Source: three-view drawing plus pictorial views. Frame: mm from the lowest corner of the part. A direction names the side the tool comes from. Round coordinates to 2 decimals unless told otherwise and drop trailing zeros. Write each loop counter-clockwise with the first axis right and the second up, starting at its lowest first coordinate (ties: lowest second). Pieces come first, ordered by that corner, then holes. Notation, with made-up numbers: M -2,-5.5 L 49,-5.5 A24 cw 49,4.5 Z; hole C 51.5,-26 d5. An arc over 180 degrees is marked long. Put each result on its own line as item: value. Start each with the question number.
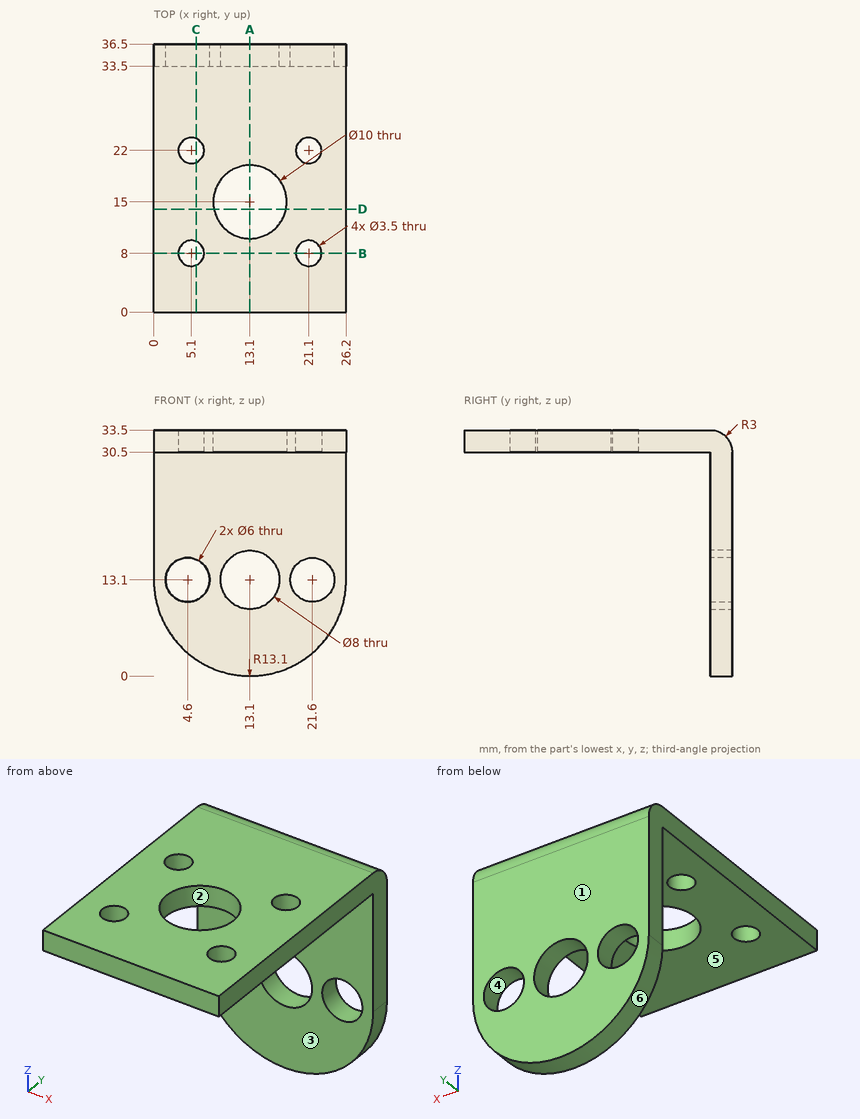
(1) Ray query, line 1 along Y through (x, z) = (18.25, 5.5); line 2 along Y through (x, z) = (5.1, 32.85); line 3 along Y through (x, z) = (5.1, 32.1). Return the intervals inside material, ascending.
(2) Access query for the marked faces 5 and 6. Directions: +Z, -Z, +X, -X, +Y, -Y. A direction counts if a zero-diameter tool reaches every point of the face in a straight line with its end or side. Return the directions, or none.
(3) Section query C-C (x = 5.75). Return loops of the section in (y, z).
(4) Pull-direction query (Y, two-part tool) for the marked faces 1, 2, 3 and 4; classes: +Y half, -Y half, draft (parallel to the pull), parting line (faces both ways), or undercut.
(5) Section query A-A (x = 13.1). Return loops of the section in (y, z).
(6) Contact query for flat-ended pins moving along their axis: P1, Ø5, axis at x = 8.5, z = 23, coming from the -Y side; P2, Ø2, axis at x = 22, z = 11.5, coming from the +Y side; P3, Ø4.5, axis at x = 21.1, y = 22, coming from the -Z side. Output: stop coordinate, or through.
(7) Section query B-B (y = 8). Return loops of the section in (x, z).
(8) Section query D-D (y = 14). Return loops of the section in (x, z), and give its area (3 significant figures).
Entries:
1. line 1: 33.5 to 36.5
1. line 2: 0 to 6.25, 9.75 to 20.25, 23.75 to 35.36
1. line 3: 0 to 6.25, 9.75 to 20.25, 23.75 to 36.04
2. face 5: -Z, +X, -X, -Y
2. face 6: -Z, +Y, -Y
3. outline: M 0,30.5 L 6.38,30.5 L 6.38,33.5 L 0,33.5 Z; M 9.62,30.5 L 20.38,30.5 L 20.38,33.5 L 9.62,33.5 Z; M 23.62,30.5 L 33.5,30.5 L 33.5,15.87 L 36.5,15.87 L 36.5,30.5 A3 ccw 33.5,33.5 L 23.62,33.5 Z; M 33.5,2.26 L 36.5,2.26 L 36.5,10.33 L 33.5,10.33 Z
4. face 1: +Y half
4. face 2: undercut
4. face 3: -Y half
4. face 4: draft
5. outline: M 0,30.5 L 10,30.5 L 10,33.5 L 0,33.5 Z; M 20,30.5 L 33.5,30.5 L 33.5,17.1 L 36.5,17.1 L 36.5,30.5 A3 ccw 33.5,33.5 L 20,33.5 Z; M 33.5,0 L 36.5,0 L 36.5,9.1 L 33.5,9.1 Z
6. P1: y = 33.5
6. P2: through
6. P3: z = 30.5
7. outline: M 0,30.5 L 3.35,30.5 L 3.35,33.5 L 0,33.5 Z; M 6.85,30.5 L 19.35,30.5 L 19.35,33.5 L 6.85,33.5 Z; M 22.85,30.5 L 26.2,30.5 L 26.2,33.5 L 22.85,33.5 Z
8. outline: M 0,30.5 L 8.2,30.5 L 8.2,33.5 L 0,33.5 Z; M 18,30.5 L 26.2,30.5 L 26.2,33.5 L 18,33.5 Z
8. area: 49.2 mm2
